Autodesk Inventor part; units mm, degrees
ref_plane "IP1_XY" through (0, 0, 0) normal (1, 0, 0) x (0, 0, -1)
ref_plane "IP1_YZ" through (0, 0, 0) normal (0, 0, -1) x (0, 1, 0)
ref_plane "IP1_ZX" through (0, 0, 0) normal (0, 1, 0) x (1, 0, 0)
sketch "Sketch_1" plane through (0, 0, 0) normal (0, 0, 1) x (1, 0, 0)
  line L0 (2.6667, 0) -> (20, 0)
  line L1 (20, 0) -> (20, -6)
  line L2 (20, -6) -> (17, -9)
  line L3 (17, -9) -> (0.8854, -9)
  line L4 (0.8854, -9) -> (0, -7.4665)
  line L5 (0, -7.4665) -> (0, -4.6188)
  line L6 (0, -4.6188) -> (2.6667, 0)
  line L7 (2.6667, 0) -> (20, 0)
revolve "Revolution1" add sketch "Sketch_1" angle 360 about axis through (2.6667, 0, 0) along (1, 0, 0)
thread "Thread1"
sketch "Sketch_2" plane through (0, 0, 0) normal (1, 0, 0) x (0, 1, 0)
  line L0 (0, 4.6188) -> (-4, 2.3094)
  line L1 (-4, 2.3094) -> (-4, -2.3094)
  line L2 (-4, -2.3094) -> (0, -4.6188)
  line L3 (0, -4.6188) -> (4, -2.3094)
  line L4 (4, -2.3094) -> (4, 2.3094)
  line L5 (4, 2.3094) -> (0, 4.6188)
extrude "Extrusion1" cut sketch "Sketch_2" along normal blind 10
ref_plane "IP1_XY" through (0, 0, 0) normal (1, 0, 0) x (0, 0, -1)
ref_plane "IP1_YZ" through (0, 0, 0) normal (0, 0, -1) x (0, 1, 0)
ref_plane "IP1_ZX" through (0, 0, 0) normal (0, 1, 0) x (1, 0, 0)
ref_plane "IP2_XY" through (20, 0, 0) normal (1, 0, 0) x (0, 0, -1)
ref_plane "IP2_YZ" through (20, 0, 0) normal (0, 0, -1) x (0, 1, 0)
ref_plane "IP2_ZX" through (20, 0, 0) normal (0, 1, 0) x (1, 0, 0)
properties part number "DIN-913 - M18x20"
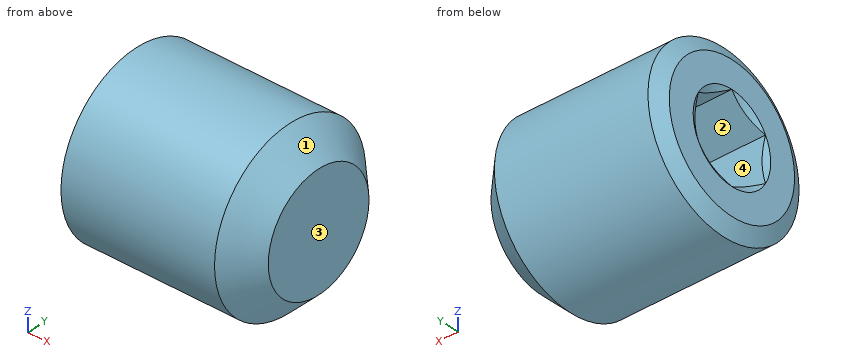
The listing builds one solid part. Answer for the finished solid, in the listing's coordinates (mm). Face numbers are marked on the shaded views. Give positions to 0.01 mm unless a question says otherwise; leave off trailing zeros. Order: outer loops, then holes, each group sorted by start corner. A loop starts at its lowest first (then second) coordinate and runs counter-clockwise, first axis right, second up. Notation, with made-up numbers: (51.5, 75) - (86.5, 75) arc R35 cw to (86.5, 109) - close; hole circle Ø1 at (-7.75, 74.5). An arc over 180 degrees is marked (long way). One line per item, written item: value. Start each with the question number.
1) A cutting plane is placed at A-A on x = 7.5. Give the vertices of the cut face in (y, z), then the cut area to 3 significant figures.
2) Given pin 1 Ø3 at (x, y) = (5.5, 5) entering from +Z; pin 2 Ø5 at (x, z) = (16, -6.5) entering from +Y; pin 3 Ø2.5 at (y, z) = (-2, 1.5) entering from -X, each flat-ended and moving along its own axis, determine where each tip first touches the part or whether it passes through.
3) Find the intervals of material crossed by L1, parallel to Z at x = 1, y = 1; L2, parallel to X at y = 3, z = -0.5; L3, parallel to Z at x = 8, y = 2.75, in increasing order.
4) A cutting plane is placed at D-D on x = 15. Give the vertices of the cut face in (y, z).
5) A cutting plane is placed at C-C on x = 17.75. Give the vertices of the cut face in (y, z), then the cut area to 3 significant figures.
6) The mould has two halves that part along Z. Classify the marked faces 1, 2, 3 and 4: released by +Z, released by -Z, zero draft, split by the parting line, or undercut.
7) A cutting plane is placed at B-B on z = 0. Give the vertices of the cut face in (x, y).
Answer sheet:
1. outline: circle Ø18 at (0, 0); hole (-4, -2.31) - (0, -4.62) - (4, -2.31) - (4, 2.31) - (0, 4.62) - (-4, 2.31) - close
1. area: 199 mm2
2. pin 1: stops at z = 8.29
2. pin 2: stops at y = 8.06
2. pin 3: stops at x = 10
3. L1: z = -8.94 to -4.04, 4.04 to 8.94
3. L2: x = 10 to 20
3. L3: z = -8.57 to -3.03, 3.03 to 8.57
4. outline: circle Ø18 at (0, 0)
5. outline: circle Ø16.5 at (0, 0)
5. area: 214 mm2
6. face 1: split by the parting line
6. face 2: undercut
6. face 3: zero draft
6. face 4: undercut
7. outline: (0, -7.47) - (0.89, -9) - (17, -9) - (20, -6) - (20, 6) - (17, 9) - (0.89, 9) - (0, 7.47) - (0, 4.62) - (0.36, 4) - (10, 4) - (10, -4) - (0.36, -4) - (0, -4.62) - close
